```python
from build123d import *

# Parameters (mm, degrees)
ESBO_O3_W                = 100
ESBO_O3_H                = 60
RESSALTO_EXTRUS_O1_DEPTH = 55
ESBO_O4_W                = 90
ESBO_O4_H                = 54
CORTE_EXTRUS_O1_DEPTH    = 45
ESBO_O5_R                = 5
CORTE_EXTRUS_O2_DEPTH    = 100
FILETE1_R                = 10


with BuildPart() as part:
    # Esboço3 → Ressalto-extrusão1 (new body)
    with BuildSketch(Plane(origin=(0, 0, 0), x_dir=(1, 0, 0), z_dir=(0, 1, 0))):
        Rectangle(ESBO_O3_W, ESBO_O3_H)
    extrude(amount=RESSALTO_EXTRUS_O1_DEPTH)

    # Esboço4 → Corte-extrusão1 (cut)
    with BuildSketch(Plane(origin=(0, 55, 0), x_dir=(1, 0, 0), z_dir=(0, 1, 0))):
        Rectangle(ESBO_O4_W, ESBO_O4_H)
    extrude(amount=-CORTE_EXTRUS_O1_DEPTH, mode=Mode.SUBTRACT)

    # Esboço5 → Corte-extrusão2 (cut)
    with BuildSketch(Plane(origin=(50, 0, 0), x_dir=(0, 0, -1), z_dir=(1, 0, 0))):
        with Locations((0, 35)):
            Circle(ESBO_O5_R)
    extrude(amount=-CORTE_EXTRUS_O2_DEPTH, mode=Mode.SUBTRACT)

    # Filete1
    filete1_edges = [part.edges().sort_by_distance(p)[0] for p in [
        (-45, 32.5, 27),
        (-45, 32.5, -27),
        (45, 32.5, -27),
        (45, 32.5, 27),
        (-50, 27.5, -30),
        (50, 27.5, -30),
        (50, 27.5, 30),
        (-50, 27.5, 30),
    ]]
    fillet(filete1_edges, radius=FILETE1_R)


solid = part.part
```
The model under review builds one solid part; all positions refer to its coordinate system, in mm. A direction names the side the tool comes from. Coordinates: 2 decimals unless noted, no trailing zeros. Order: outer loops, then holes, each group sorted by start corner. A loop starts at its lowest first (then second) coordinate and runs counter-clockwise, first axis right, second up. Notation, with made-up numbers: (40, 48) -> (70, 48) arc R15 cw to (70, 54) -> close; hole circle Ø1 at (29, -6.5). An arc over 180 degrees is marked (long way). Answer in a Markdown table with one row per item. Add a question column.
Item 1: Machinability: for faces 4 (the cylindrical face through (-47.15, 27.88, -26.99)), 5 (the cylindrical face through (-41.99, 32.18, 24.15)), which of the approach directions +Z, -Z, +X, -X, +Y, -Y give a long, thin tool a straight path to every point of the face, cutting with its end or side? Answer none if there is none.
Item 2: Mouldability with a two-part tool opening along Y and no side actions: class faces 1 (the cylindrical face through (-47, 39, -3)), 2 (the flat face through (0, 33, -27)), 3 (the flat face through (-1, 10, 0)) as +Y half, -Y half, draft (parallel to the pull), parting line (faces both ways), or undercut.
Item 3: To check wall thickness, follow probe 1 along Z at (x, y) = (-1, 30.5); probe 2 along X at (y, z) = (13, -6.5); probe 3 along Y at (x, z) = (-47, 0). State the ranges of each line that lie inside material, in increasing order.
Item 4: We need section A-A on y = 35. Write out the cut boundary in (x, z), plus the area to 3 significant figures.
Item 5: We need section C-C on y = 26.5. Write out the cut boundary in (x, z), plus the area to 3 significant figures.
Item 6: We need section D-D on x = 7.5. Write out the cut boundary in (y, z).
Item 7: Clearance check with a flat-ended pin moving along its axis: pin 1 (12 mm diameter, centred on x = 34.5, z = -0.5, fed in from +Y). State where the tip first meets the part, or that it passes through.
Item 8: We need section B-B on z = 0. Write out the cut boundary in (x, y).
Final values:
| question | item | result |
|---|---|---|
| 1 | face 4 | -Z, -X, +Y, -Y |
| 1 | face 5 | +Y |
| 2 | face 1 | undercut |
| 2 | face 2 | draft |
| 2 | face 3 | +Y half |
| 3 | probe 1 | z = -30 to -27, 27 to 30 |
| 3 | probe 2 | x = -50 to -45, 45 to 50 |
| 3 | probe 3 | y = 0 to 30, 40 to 55 |
| 4 | outline | (-50, -20) arc R10 ccw to (-40, -30) -> (40, -30) arc R10 ccw to (50, -20) -> (50, -5) -> (45, -5) -> (45, -17) arc R10 cw to (35, -27) -> (-35, -27) arc R10 cw to (-45, -17) -> (-45, -5) -> (-50, -5) -> close; (-50, 5) -> (-45, 5) -> (-45, 17) arc R10 cw to (-35, 27) -> (35, 27) arc R10 cw to (45, 17) -> (45, 5) -> (50, 5) -> (50, 20) arc R10 ccw to (40, 30) -> (-40, 30) arc R10 ccw to (-50, 20) -> close |
| 4 | area | 1,040 mm2 |
| 5 | outline | (-50, -20) arc R10 ccw to (-40, -30) -> (40, -30) arc R10 ccw to (50, -20) -> (50, 20) arc R10 ccw to (40, 30) -> (-40, 30) arc R10 ccw to (-50, 20) -> close; hole (-45, -17) arc R10 ccw to (-35, -27) -> (35, -27) arc R10 ccw to (45, -17) -> (45, 17) arc R10 ccw to (35, 27) -> (-35, 27) arc R10 ccw to (-45, 17) -> close |
| 5 | area | 1,140 mm2 |
| 6 | outline | (0, -30) -> (55, -30) -> (55, -27) -> (10, -27) -> (10, 27) -> (55, 27) -> (55, 30) -> (0, 30) -> close |
| 7 | pin 1 | stops at y = 10 |
| 8 | outline | (-50, 0) -> (50, 0) -> (50, 30) -> (45, 30) -> (45, 10) -> (-45, 10) -> (-45, 30) -> (-50, 30) -> close; (-50, 40) -> (-45, 40) -> (-45, 55) -> (-50, 55) -> close; (45, 40) -> (50, 40) -> (50, 55) -> (45, 55) -> close |
